Design review of the part built by this model. Coordinates are the model's own, in mm. A direction names the side the tool comes from. Round coordinates to 2 decimals unless told otherwise and drop trailing zeros. Loops run counter-clockwise (first coordinate to the right, second up) from the corner with the lowest first, then second, coordinate; pieces in that order, holes last. Notation, with made-up numbers: (60.25, 54.25) - (97.25, 54.25) arc R23 cw to (97.25, 90.25) - close; hole circle Ø1 at (-30, -24.75). An arc over 180 degrees is marked (long way). Return JSON: item names as keys, results as strings. Group by question number.
(1) Clearance check with flat-ended pins moving along their axes: pin 1 (5 mm diameter, centred on x = -8.75, z = 10, fed in from +Y); pin 2 (1.7 mm diameter, centred on x = 8.5, z = 5.5, fed in from +Y); pin 3 (1.2 mm diameter, centred on x = -9.5, y = -48, fed in from -Z); pin 4 (3 mm diameter, centred on y = -15, z = 10, fed in from +X). State where each tip first meets the part, or that it passes through.
(2) Wall thickness on L1, parallel to X at y = -48.5, z = 10.25; L2, parallel to Z at x = 8.75, y = -42; L3, parallel to X at y = -15, z = 19: over which ranges is each line inside the solid? List them lowest first. Write a range as [from, to].
(3) We need section D-D, the plane z = 16. Write out the cut boundary in (x, y).
(4) The part is to be moulded in two halves that separate along Z. For faces 5 (the flat face through (13.535, -16.901, 13.232)), 6 (the flat face through (6, -53.594, 10)), 7 (the flat face through (-3, -18, 0)), 8 (the cylindrical face through (7.276, -52.18, 11.352)), say which applies: pulls with the +Z half, pulls with the -Z half, needs draft (parallel to the pull), parting line crosses it, or undercut.
(5) We need section B-B, the plane x = 8.75. Write out the cut boundary in (y, z), and give its area (3 significant figures).
(6) For faces 1 (the flat face through (14, -11.25, 10)), 2 (the cylindrical face through (10.658, -42.717, 10.601)), 3 (the flat face through (1.5, -14, 12)), 4 (the flat face through (9, -49, 15)), list the 3-axis set-ups (+Z, -Z, +X, -X, +Y, -Y) from which the entire face can be reached by the end or side of a thin tool; tool diameter is ignored.
(7) We need section C-C, the plane y = -4.5. Write out the cut boundary in (x, z), and give its area (3 significant figures).
(8) We need section A-A, the plane z = 2.5. Write out the cut boundary in (x, y).
from build123d import *

# Parameters (mm, degrees)
PAD_DEPTH       = 20
SKETCH004_R     = 1.75
POCKET002_DEPTH = 50
POCKET003_DEPTH = 5
POCKET004_DEPTH = 15
SKETCH007_R     = 2
POCKET005_DEPTH = 15
SKETCH008_R     = 8.1
POCKET006_DEPTH = 10


with BuildPart() as part:
    # Sketch003 → Pad (new body)
    with BuildSketch(Plane.XY):
        with BuildLine():
            Line((-8, -26.6), (-8, -40.1))
            ThreePointArc((-8, -40.1), (-5.061117, -42.425857), (-1.5, -43.594227))
            Line((-1.5, -53.594227), (-1.5, -43.594227))
            Line((-13.5, -53.594227), (-1.5, -53.594227))
            ThreePointArc((-16, -51.094227), (-15.267767, -52.861994), (-13.5, -53.594227))
            Line((-16, 0), (-16, -51.094227))
            ThreePointArc((16, 0), (0, 16), (-16, 0))
            Line((16, -51.094227), (16, 0))
            ThreePointArc((13.5, -53.594227), (15.267767, -52.861994), (16, -51.094227))
            Line((1.5, -53.594227), (13.5, -53.594227))
            Line((1.5, -53.594227), (1.5, -43.594227))
            ThreePointArc((1.5, -43.594227), (5.061117, -42.425857), (8, -40.1))
            Line((8, -40.1), (8, -26.6))
            ThreePointArc((8, -26.6), (5.061117, -24.274143), (1.5, -23.105773))
            Line((1.5, -5.809475), (1.5, -23.105773))
            ThreePointArc((1.5, -5.809475), (0, 6), (-1.5, -5.809475))
            Line((-1.5, -5.809475), (-1.5, -23.105773))
            ThreePointArc((-1.5, -23.105773), (-5.061117, -24.274143), (-8, -26.6))
        make_face()
    extrude(amount=PAD_DEPTH)

    # Sketch004 (on Face9 of Pad) → Pocket002 (cut)
    with BuildSketch(Plane(origin=(-16, 0, 0), x_dir=(0, -1, 0), z_dir=(-1, 0, 0))):
        with Locations((15, 10)):
            Circle(SKETCH004_R)
    extrude(amount=-POCKET002_DEPTH, mode=Mode.SUBTRACT)

    # Sketch005 (on Face17 of Pocket002) → Pocket003 (cut)
    with BuildSketch(Plane(origin=(16, 0, 0), x_dir=(0, -1, 0), z_dir=(-1, 0, 0))):
        Polygon((18.75, 7.834936), (18.75, 12.165064), (15, 14.330127), (11.25, 12.165064), (11.25, 7.834936), (15, 5.669873), align=None)
    extrude(amount=POCKET003_DEPTH, mode=Mode.SUBTRACT)

    # Sketch006 → Pocket004 (cut)
    with BuildSketch(Plane(origin=(0, 0, 0), x_dir=(1, 0, 0), z_dir=(0, 0, -1))):
        Polygon((-7, 50.72662), (-6.15, 50.72662), (-6.15, 46.72662), (-11.85, 46.72662), (-11.85, 50.72662), (-11, 50.72662), align=None)
        Polygon((11, 50.72662), (11.85, 50.72662), (11.85, 46.72662), (6.15, 46.72662), (6.15, 50.72662), (7, 50.72662), align=None)
    extrude(amount=-POCKET004_DEPTH, mode=Mode.SUBTRACT)

    # Sketch007 (on Face16 of Pocket004) → Pocket005 (cut)
    with BuildSketch(Plane.XZ.offset(53.594227)):
        with Locations((-8.75, 10)):
            Circle(SKETCH007_R)
        with Locations((8.75, 10)):
            Circle(SKETCH007_R)
    extrude(amount=-POCKET005_DEPTH, mode=Mode.SUBTRACT)

    # Sketch008 (on Face4 of Pocket005) → Pocket006 (cut)
    with BuildSketch(Plane(origin=(0, 0, 0), x_dir=(1, 0, 0), z_dir=(0, 0, -1))):
        Circle(SKETCH008_R)
    extrude(amount=-POCKET006_DEPTH, mode=Mode.SUBTRACT)


solid = part.part
Solutions:
{
 "1": {"pin 1": "y = 14.73", "pin 2": "y = 14.05", "pin 3": "z = 15", "pin 4": "through"},
 "2": {"L1": "[-16, -11.85], [-6.15, -1.5], [1.5, 6.15], [11.85, 16]", "L2": "[0, 8], [12, 20]", "L3": "[-16, -1.5], [1.5, 16]"},
 "3": {"outline": "(-16, -51.09) arc R2.5 ccw to (-13.5, -53.59) - (-1.5, -53.59) - (-1.5, -43.59) arc R10.69 cw to (-8, -40.1) - (-8, -26.6) arc R10.69 cw to (-1.5, -23.11) - (-1.5, -5.81) arc R6 cw (long way) to (1.5, -5.81) - (1.5, -23.11) arc R10.69 cw to (8, -26.6) - (8, -40.1) arc R10.69 cw to (1.5, -43.59) - (1.5, -53.59) - (13.5, -53.59) arc R2.5 ccw to (16, -51.09) - (16, 0) arc R16 ccw to (-16, 0) - close"},
 "4": {"face 5": "undercut", "face 6": "needs draft", "face 7": "pulls with the -Z half", "face 8": "undercut"},
 "5": {"outline": "(-53.59, 0) - (-50.73, 0) - (-50.73, 8) - (-53.59, 8) - close; (-53.59, 12) - (-50.73, 12) - (-50.73, 15) - (-46.73, 15) - (-46.73, 12) - (-38.59, 12) - (-38.59, 8) - (-46.73, 8) - (-46.73, 0) - (13.4, 0) - (13.4, 20) - (-53.59, 20) - close; hole circle Ø3.5 at (-15, 10)", "area": "1,230 mm^2"},
 "6": {"face 1": "+X", "face 2": "-Y", "face 3": "+Z, -Z, -Y", "face 4": "-Z"},
 "7": {"outline": "(-16, 0) - (-6.73, 0) - (-6.73, 10) - (-3.97, 10) - (-3.97, 20) - (-16, 20) - close; (3.97, 10) - (6.73, 10) - (6.73, 0) - (16, 0) - (16, 20) - (3.97, 20) - close", "area": "426 mm^2"},
 "8": {"outline": "(-16, -51.09) arc R2.5 ccw to (-13.5, -53.59) - (-1.5, -53.59) - (-1.5, -43.59) arc R10.69 cw to (-8, -40.1) - (-8, -26.6) arc R10.69 cw to (-1.5, -23.11) - (-1.5, -7.96) arc R8.1 cw (long way) to (1.5, -7.96) - (1.5, -23.11) arc R10.69 cw to (8, -26.6) - (8, -40.1) arc R10.69 cw to (1.5, -43.59) - (1.5, -53.59) - (13.5, -53.59) arc R2.5 ccw to (16, -51.09) - (16, 0) arc R16 ccw to (-16, 0) - close; hole (-11.85, -50.73) - (-6.15, -50.73) - (-6.15, -46.73) - (-11.85, -46.73) - close; hole (6.15, -50.73) - (11.85, -50.73) - (11.85, -46.73) - (6.15, -46.73) - close"}
}
